```python
from build123d import *

# Parameters (mm, degrees)
F0_W     = 31.75
F0_H     = 77.724
F1_DEPTH = 14.224
F2_DEPTH = 7.874
F4_DEPTH = 88.901
F5_DEPTH = 12.7


with BuildPart() as f1:
    # F0 (on Top) → F1 (new body, symmetric)
    with BuildSketch(Plane.XY):
        Rectangle(F0_W, F0_H)
    extrude(amount=F1_DEPTH, both=True)

    # F0 (on Top) → F2 (join, symmetric)
    with BuildSketch(Plane.XY):
        Polygon((-15.875, -38.862), (-15.875, 38.862), (-44.45, 38.862), (-44.45, -30.734), (-26.924, -30.734), (-26.924, -52.577469), (-15.875, -41.528469), align=None)
        with BuildLine():
            Line((-35.814, -15.24), (-35.814, 8.636))
            ThreePointArc((-35.814, 8.636), (-30.226, 14.224), (-24.638, 8.636))
            Line((-24.638, 8.636), (-24.638, -15.24))
            ThreePointArc((-24.638, -15.24), (-30.226, -20.828), (-35.814, -15.24))
        make_face(mode=Mode.SUBTRACT)
        Polygon((44.45, 38.862), (15.875, 38.862), (15.875, -38.862), (15.875, -41.528469), (26.924, -52.577469), (26.924, -30.734), (44.45, -30.734), align=None)
        with BuildLine():
            ThreePointArc((24.638, 8.636), (30.226, 14.224), (35.814, 8.636))
            Line((35.814, 8.636), (35.814, -15.24))
            ThreePointArc((35.814, -15.24), (30.226, -20.828), (24.638, -15.24))
            Line((24.638, -15.24), (24.638, 8.636))
        make_face(mode=Mode.SUBTRACT)
    extrude(amount=F2_DEPTH, both=True)

    # F3 (on face) → F4 (cut, through all)
    with BuildSketch(Plane(origin=(-44.45, 0, 0), x_dir=(0, -1, 0), z_dir=(-1, 0, 0))):
        Polygon((-38.862, 7.874), (-38.862, 3.048), (-32.512, 3.048), (-32.512, 17.1704), (-38.862, 17.1704), align=None)
    extrude(amount=-F4_DEPTH, mode=Mode.SUBTRACT)

    # F0 (on Top) → F5 (join, symmetric)
    with BuildSketch(Plane.XY):
        Polygon((-26.924, -30.734), (-44.45, -30.734), (-44.45, -65.786), (-40.132531, -65.786), (-30.353265, -56.006734), (-26.924, -52.577469), align=None)
        Polygon((44.45, -65.786), (44.45, -30.734), (26.924, -30.734), (26.924, -52.577469), (30.353265, -56.006733), (40.132531, -65.786), align=None)
    extrude(amount=F5_DEPTH, both=True)


solid = f1.part
```
Geometry: final body of the model. Coordinates: model frame, mm. A direction names the side the tool comes from. Round coordinates to 2 decimals unless told otherwise and drop trailing zeros. Write each loop counter-clockwise with the first axis right and the second up, starting at its lowest first coordinate (ties: lowest second). Pieces come first, ordered by that corner, then holes. Notation, with made-up numbers: M 78.5,-1 L 121.5,-1 A31 cw 121.5,33 Z; hole C 56.25,73.25 d1. An arc over 180 degrees is marked long. Answer in a Markdown table with one row per item. Add a question column.
(1) Cut plane B-B, the plane y = -9. Return the cut outline in (x, z) (3 decimals).
(2) Reachability of faces 5 (the face through (35.814, -3, 0)), 6 (the face through (0, -38.862, 0)), 7 (the face through (-36, -44, 12.7)), 8 (the face through (-44.45, -24, 0)), 9 (the face through (-36, -30.734, -10)) from +Z, -Z, +X, -X, +Y, -Y: full face, straight path, thin tool, end or side. Return the list, or none.
(3) Cut plane C-C, the plane z = 0.75. Return the cut outline in (x, y) (3 decimals).
(4) Ray query, L1, parallel to X at y = -1, z = 1.75; L2, parallel to X at y = -20, z = -4.25; L3, parallel to Z at x = -17, y = 33. Return the intervals inside material, ascending.
(5) Cut plane A-A, the plane y = -40. Return the cut outline in (x, z) (3 decimals).
(6) Cut plane D-D, the plane z = -9.5. Return the cut outline in (x, y) (3 decimals), then the cut area to 3 significant figures.
(7) Contact query for flat-ended pins moving along their axis: pin 1 (7 mm diameter, centred on y = 14, z = 11.5, fed in from +X) (3 decimals); pin 2 (4 mm diameter, centred on x = -19.5, z = 3, fed in from -Y); pin 3 (19.5 mm diameter, centred on x = -34.5, y = -49, fed in from -Z). Output: stop coordinate, or through.
(8) Draft query along Y for faces 1 (the face through (-36, -44, -12.7)), 2 (the face through (-24.638, -3, 0)), 3 (the face through (-30.103, -20.827, -0.11)), 4 (the face through (-1, 32.512, 7)). Return one class per face: pulls with the +Y half, pulls with the -Y half, needs draft (parallel to the pull), parting line crosses it, or undercut.
Established:
| question | item | result |
|---|---|---|
| 1 | outline | M -44.45,-7.874 L -35.814,-7.874 L -35.814,7.874 L -44.45,7.874 Z; M -24.638,-7.874 L -15.875,-7.874 L -15.875,-14.224 L 15.875,-14.224 L 15.875,-7.874 L 24.638,-7.874 L 24.638,7.874 L 15.875,7.874 L 15.875,14.224 L -15.875,14.224 L -15.875,7.874 L -24.638,7.874 Z; M 35.814,-7.874 L 44.45,-7.874 L 44.45,7.874 L 35.814,7.874 Z |
| 2 | face 5 | +Z, -Z |
| 2 | face 6 | +Z, -Z, -Y |
| 2 | face 7 | +Z, -X, +Y, -Y |
| 2 | face 8 | +Z, -Z, -X, +Y, -Y |
| 2 | face 9 | -Z, -X, +Y |
| 3 | outline | M -44.45,-65.786 L -40.133,-65.786 L -15.875,-41.528 L -15.875,-38.862 L 15.875,-38.862 L 15.875,-41.528 L 26.924,-52.577 L 30.353,-56.007 L 40.133,-65.786 L 44.45,-65.786 L 44.45,38.862 L -44.45,38.862 Z; hole M -35.814,-15.24 A5.588 ccw -24.638,-15.24 L -24.638,8.636 A5.588 ccw -35.814,8.636 Z; hole M 24.638,-15.24 A5.588 ccw 35.814,-15.24 L 35.814,8.636 A5.588 ccw 24.638,8.636 Z |
| 4 | L1 | -44.45 to -35.81, -24.64 to 24.64, 35.81 to 44.45 |
| 4 | L2 | -44.45 to -33.15, -27.3 to 27.3, 33.15 to 44.45 |
| 4 | L3 | -7.87 to 3.05 |
| 5 | outline | M -44.45,-12.7 L -26.924,-12.7 L -26.924,-7.874 L -15.875,-7.874 L -15.875,7.874 L -26.924,7.874 L -26.924,12.7 L -44.45,12.7 Z; M 15.875,-7.874 L 26.924,-7.874 L 26.924,-12.7 L 44.45,-12.7 L 44.45,12.7 L 26.924,12.7 L 26.924,7.874 L 15.875,7.874 Z |
| 6 | outline | M -44.45,-65.786 L -40.133,-65.786 L -26.924,-52.577 L -26.924,-30.734 L -44.45,-30.734 Z; M -15.875,-38.862 L 15.875,-38.862 L 15.875,38.862 L -15.875,38.862 Z; M 26.924,-52.577 L 30.353,-56.007 L 40.133,-65.786 L 44.45,-65.786 L 44.45,-30.734 L 26.924,-30.734 Z |
| 6 | area | 3,520 mm² |
| 7 | pin 1 | x = 15.875 |
| 7 | pin 2 | y = -47.15 |
| 7 | pin 3 | z = -12.7 |
| 8 | face 1 | needs draft |
| 8 | face 2 | undercut |
| 8 | face 3 | undercut |
| 8 | face 4 | pulls with the +Y half |
